Geometry check sheet. Reference: the model listing, model coordinates, mm. A direction names the side the tool comes from. Coordinates: 2 decimals unless noted, no trailing zeros. Write each loop counter-clockwise with the first axis right and the second up, starting at its lowest first coordinate (ties: lowest second). Pieces come first, ordered by that corner, then holes. Notation, with made-up numbers: M 63,-29.75 L 75,-29.75 A14 ccw 75,-12.75 Z; hole C 29.25,-27.5 d9. An arc over 180 degrees is marked long. Answer as a JSON object with one key per item and string values. Group by question number.
Autodesk Inventor part; units mm, degrees
ref_plane "YZ Plane" through (0, 0, 0) normal (1, 0, 0) x (0, 1, 0)
ref_plane "XZ Plane" through (0, 0, 0) normal (0, 1, 0) x (-1, 0, 0)
ref_plane "XY Plane" through (0, 0, 0) normal (0, 0, 1) x (1, 0, 0)
sketch "Sketch1" plane through (0, 0, 0) normal (0, 1, 0) x (-1, 0, 0)
  line L0 (0, 0) -> (0, -81.8644)
  line L1 (4.678, -40.9322) -> (4.678, 5.8475)
  line L2 (4.678, -40.9322) -> (4.678, -87.7119)
  line L3 (4.678, 5.8475) -> (-64.322, 5.8475)
  line L4 (-64.322, 5.8475) -> (-64.322, 0)
  line L5 (-64.322, 0) -> (0, 0)
  line L6 (0, -81.8644) -> (-64.322, -81.8644)
  line L7 (-64.322, -81.8644) -> (-64.322, -87.7119)
  line L8 (-64.322, -87.7119) -> (4.678, -87.7119)
  dimension "d4" = 69
extrude "Extrusion1" add sketch "Sketch1" along normal blind 25.4
sketch "Sketch2" plane through (-4.678, 0, -87.7119) normal (-1, 0, 0) x (0, 0, 1)
  line L0 (87.7119, 25.4) -> (5.8475, 25.4)
  line L1 (87.7119, 0) -> (5.8475, 0)
  line L2 (40, -8.93) -> (50.35, -8.93)
  line L3 (50.35, -8.93) -> (53.35, -8.93)
  line L4 (40, -8.93) -> (29.65, -8.93)
  line L5 (29.65, -8.93) -> (26.65, -8.93)
  line L6 (53.35, -8.93) -> (53.35, 25.4)
  line L7 (26.65, -8.93) -> (26.65, 25.4)
  line L8 (26.65, 25.4) -> (53.35, 25.4)
  dimension "d19" = 3
  dimension "d20" = 10.35
  dimension "d26" = 34.33
extrude "Extrusion2" add sketch "Sketch2" along normal blind 46
sketch "Sketch3" plane through (0, 25.4, 0) normal (0, 1, 0) x (1, 0, 0)
  line L0 (-50.678, 34.3619) -> (-50.678, 61.0619)
  line L1 (-50.678, 47.7119) -> (-50.678, 58.0619)
  line L2 (-50.678, 47.7119) -> (-50.678, 37.3619)
  line L3 (-50.678, 58.0619) -> (-4.678, 58.0619)
  line L4 (-4.678, 61.0619) -> (-4.678, 34.3619)
  line L5 (-4.678, 58.0619) -> (-4.678, 37.3619)
  line L6 (-4.678, 37.3619) -> (-50.678, 37.3619)
  point P0 (0, 0)
  dimension "d24" = 10.35
  dimension "d25" = 10.35
extrude "Extrusion3" cut sketch "Sketch3" against normal blind 31.33
sketch "Sketch4" plane through (0, -5.93, 0) normal (0, 1, 0) x (1, 0, 0)
  line L0 (-50.678, 61.0619) -> (-50.678, 34.3619)
  line L1 (-33.878, 47.7119) -> (-33.878, 58.0619)
  line L2 (-50.678, 58.0619) -> (-4.678, 58.0619)
  line L3 (-33.878, 58.0619) -> (-26.878, 58.0619)
  line L4 (-26.878, 58.0619) -> (-26.878, 37.3619)
  line L5 (-4.678, 37.3619) -> (-50.678, 37.3619)
  line L6 (-26.878, 37.3619) -> (-33.878, 37.3619)
  line L7 (-33.878, 37.3619) -> (-33.878, 47.7119)
  point P0 (0, 0)
  dimension "d30" = 7
extrude "Extrusion4" add sketch "Sketch4" along normal blind 6 contours L2 L4 L5 L7 L1
sketch "Sketch5" plane through (-33.878, -5.93, -58.0619) normal (-1, 0, 0) x (0, 0, 1)
  line L0 (20.7, 0) -> (20.7, 5.93)
  line L1 (0, 6) -> (0, 0)
  circle A0 centre (5.35, 3) radius 1
  circle A1 centre (15.35, 2.965) radius 1.035
  point P0 (58.0619, 5.93)
  dimension "d35" = 2
extrude "Extrusion5" cut sketch "Sketch5" against normal through all
sketch "Sketch6" plane through (-4.678, -8.93, -34.3619) normal (0, 0, 1) x (1, 0, 0)
  line L0 (-29.2, 3) -> (-46, 3)
  line L1 (0, 0) -> (-46, 0)
  line L2 (-46, 0) -> (-51, 0)
  line L3 (-51, 0) -> (-51, 3)
  line L4 (-59, 11.315) -> (-51, 3)
  line L5 (-51, 19.63) -> (-46, 19.63)
  line L6 (-46, 0) -> (-46, 34.33)
  line L7 (69, 8.93) -> (69, 34.33)
  line L8 (-59, 11.315) -> (-89, 11.315)
  line L9 (-89, 11.315) -> (-89, 19.63)
  line L10 (-89, 19.63) -> (-51, 19.63)
  point P0 (4.678, 8.93)
  dimension "d41" = 5
  dimension "d42" = 16.63
  dimension "d46" = 30
extrude "Extrusion6" add sketch "Sketch6" against normal up to surface (26.7 mm away)
sketch "Sketch7" plane through (-93.678, 2.385, -34.3619) normal (-1, 0, 0) x (0, 0, 1)
  line L0 (-3, 8.315) -> (-23.7, 8.315)
  circle A0 centre (-13.35, 8.315) radius 3
  point P0 (34.3619, -2.385)
  point P1 (-16.35, 8.315)
  point P2 (-10.35, 8.315)
  dimension "d49" = 6
extrude "Extrusion7" cut sketch "Sketch7" against normal up to surface (43 mm away) contours A0 L0 picked at (-13.9181, 7.492)
sketch "Sketch8" plane through (-93.678, 2.385, -34.3619) normal (-1, 0, 0) x (0, 0, 1)
  arc A0 (-16.35, 8.315) -> (-10.35, 8.315) centre (-13.35, 8.315) ccw
  circle A1 centre (-13.35, 8.315) radius 6
  point P0 (34.3619, -2.385)
  dimension "d52" = 12
extrude "Extrusion8" cut sketch "Sketch8" against normal blind 10
sketch "Sketch9" plane through (-55.678, -8.93, -34.3619) normal (-1, 0, 0) x (0, 0, 1)
  circle A0 centre (-8.35, 5.965) radius 3.5
  circle A1 centre (-18.35, 6) radius 1
  circle A2 centre (-18.35, 6) radius 3.5
  point P0 (34.3619, 8.93)
  dimension "d55" = 7
  dimension "d56" = 7
extrude "Extrusion9" cut sketch "Sketch9" along normal blind 7 and the other way blind 5 contours A0 | A1 | A2
sketch "Sketch10" plane through (-4.678, 0, -87.7119) normal (1, 0, 0) x (0, 0, -1)
  line L0 (-53.35, -5.93) -> (-53.35, -8.93)
  line L1 (-50.35, 10.7) -> (-50.35, -5.93)
  line L2 (-53.35, -8.93) -> (-50.35, -8.93)
  line L3 (-50.35, -5.93) -> (-50.35, 0)
  line L4 (-50.35, 0) -> (-53.35, 0)
  line L5 (-53.35, 0) -> (-53.35, -8.93)
  line L6 (-26.65, -5.93) -> (-26.65, -8.93)
  line L7 (-29.65, -5.93) -> (-29.65, 10.7)
  line L8 (-26.65, -8.93) -> (-29.65, -8.93)
  line L9 (-29.65, -5.93) -> (-29.65, 0)
  line L10 (-29.65, 0) -> (-26.65, 0)
  line L11 (-26.65, 0) -> (-26.65, -8.93)
  line L12 (-29.65, -8.93) -> (-50.35, -8.93)
  line L13 (-50.35, 0) -> (-29.65, 0)
  line L14 (-29.65, 0) -> (-29.65, -5.93)
  line L15 (-50.35, -5.93) -> (-50.35, 0)
  point P0 (-87.7119, 0)
extrude "Extrusion10" add sketch "Sketch10" along normal up to surface (4.678 mm away)
sketch "Sketch13" plane through (0, 0, -81.8644) normal (0, 0, 1) x (1, 0, 0)
  line L0 (64.322, 0) -> (64.322, 25.4)
  circle A0 centre (51.822, 12.7) radius 5.75
  point P0 (0, 0)
  dimension "d76" = 11.5
extrude "Extrusion13" add sketch "Sketch13" along normal blind 5
sketch "Sketch14" plane through (-4.678, 0, 5.8475) normal (0, 0, 1) x (1, 0, 0)
  line L0 (69, 0) -> (69, 25.4)
  circle A0 centre (56.5, 12.7) radius 5.75
  circle A1 centre (56.5, 17.7) radius 1.5
  circle A2 centre (51.5, 12.7) radius 1.5
  circle A3 centre (56.5, 7.7) radius 1.5
  circle A4 centre (61.5, 12.7) radius 1.5
  point P0 (4.678, 0)
  dimension "d80" = 3
  dimension "d83" = 360
extrude "Extrusion14" cut sketch "Sketch14" against normal up to surface (5.8475 mm away) contours A0 A4 | A0 A4 | A1 A0 | A0 A1 | A3 A0 | A0 A3 | A2 A0 | A0 A2
ref_plane "Work Plane6" through (-60.678, -5.93, -58.0619) normal (1, 0, 0) x (0, 0, -1)
properties part number "Joint2"
1) Go/stop test with flat-tipped pins: pin 1 Ø12 at (x, z) = (18, -11.5) entering from +Y; pin 2 Ø5 at (y, z) = (0.5, -51.5) entering from +X; pin 3 Ø8.5 at (x, z) = (-67.5, -41) entering from +Y; pin 4 Ø7.5 at (x, z) = (-30.5, -48) entering from +Y. Record where each tip stops, or that it passes through.
2) Set-up check for faces 1 (the cylindrical face through (55.323, 12.766, 2.965)), 2 (the flat face through (52, 13, -76.864)), 3 (the cylindrical face through (-67.4, 7.7, -47.8)), 4 (the flat face through (-27, 10, -37.362)), 5 (the flat face through (24.9, 0, -82.2)): record each of +Z, -Z, +X, -X, +Y, -Y from which the full face is reachable in a straight line by a thin tool's end or side.
3) Section check A-A (x = 41). Record the cut outline in (y, z).
4) Material ranges on probe 1 along X at (y, z) = (17.7, 2.2); probe 2 along Z at (x, y) = (-32, 9); probe 3 along Z at (x, y) = (20, 4.5), recorded low to high. Write a range as [from, to].
5) Section check C-C (y = 23). Record the cut outline in (x, z), then the cut area to 3 significant figures.
6) Section check B-B (y = 12.7). Record the cut outline in (x, z), then the cut area to 3 significant figures.
7) Section check D-D (x = -11.5). Record the cut outline in (y, z), then the cut area to 3 significant figures.
8) Draft check along Z on faces 6 (the cylindrical face through (-55.1, 0.5, -43.2)), 7 (the flat face through (-55.678, -7, -48)), 8 (the flat face through (30, 13, -87.712)). Enter one of: +Z half, -Z half, draft (parallel to the pull), parting line (faces both ways), or undercut.
Entries:
{
 "1": {"pin 1": "through", "pin 2": "x = 0", "pin 3": "y = 10.7", "pin 4": "y = 0.07"},
 "2": {"face 1": "+Z", "face 2": "+X, +Y, -Y", "face 3": "-X, +Y", "face 4": "+Y", "face 5": "-Z, +X, -X, -Y"},
 "3": {"outline": "M 0,-87.71 L 25.4,-87.71 L 25.4,-81.86 L 0,-81.86 Z; M 0,0 L 25.4,0 L 25.4,5.85 L 0,5.85 Z"},
 "4": {"probe 1": "[-4.68, 50.32], [53.32, 64.32]", "probe 2": "[-61.06, -58.06], [-37.36, -34.36]", "probe 3": "[-87.71, -81.86], [0, 5.85]"},
 "5": {"outline": "M -50.68,-61.06 L -4.68,-61.06 L -4.68,-87.71 L 64.32,-87.71 L 64.32,-81.86 L 0,-81.86 L 0,0 L 64.32,0 L 64.32,5.85 L -4.68,5.85 L -4.68,-34.36 L -50.68,-34.36 L -50.68,-37.36 L -4.68,-37.36 L -4.68,-58.06 L -50.68,-58.06 Z", "area": "1,470 mm^2"},
 "6": {"outline": "M -50.68,-61.06 L -4.68,-61.06 L -4.68,-87.71 L 64.32,-87.71 L 64.32,-81.86 L 57.57,-81.86 L 57.57,-76.86 L 46.07,-76.86 L 46.07,-81.86 L 0,-81.86 L 0,0 L 45.32,0 L 45.32,5.85 L -4.68,5.85 L -4.68,-34.36 L -50.68,-34.36 L -50.68,-37.36 L -4.68,-37.36 L -4.68,-58.06 L -50.68,-58.06 Z; M 48.32,0 L 55.32,0 L 55.32,5.85 L 48.32,5.85 Z; M 58.32,0 L 64.32,0 L 64.32,5.85 L 58.32,5.85 Z", "area": "1,490 mm^2"},
 "7": {"outline": "M -8.93,-61.06 L 25.4,-61.06 L 25.4,-58.06 L -5.93,-58.06 L -5.93,-37.36 L 25.4,-37.36 L 25.4,-34.36 L -8.93,-34.36 Z", "area": "268 mm^2"},
 "8": {"face 6": "undercut", "face 7": "draft", "face 8": "-Z half"}
}
